from build123d import *

# Parameters (mm, degrees)
SKETCH1_R           = 20
BOSS_EXTRUDE1_DEPTH = 10
SKETCH2_R           = 1
BOSS_EXTRUDE2_DEPTH = 2
SKETCH3_R           = 1
BOSS_EXTRUDE3_DEPTH = 2
FILLET2_R           = 1


with BuildPart() as part:
    # Sketch1 → Boss-Extrude1 (new body)
    with BuildSketch(Plane(origin=(0, 0, 0), x_dir=(0, 0, -1), z_dir=(1, 0, 0))):
        Circle(SKETCH1_R)
    extrude(amount=BOSS_EXTRUDE1_DEPTH)

    # Sketch2 → Boss-Extrude2 (add)
    with BuildSketch(Plane(origin=(10, 0, 0), x_dir=(0, 0, -1), z_dir=(1, 0, 0))):
        Circle(SKETCH2_R)
    extrude(amount=BOSS_EXTRUDE2_DEPTH)

    # Sketch3 → Boss-Extrude3 (add)
    with BuildSketch(Plane.ZY):
        Circle(SKETCH3_R)
    extrude(amount=BOSS_EXTRUDE3_DEPTH)

    # Fillet2
    fillet2_edges = [part.edges().sort_by_distance(p)[0] for p in [
        (0, 0, 20),
        (10, 0, 20),
    ]]
    fillet(fillet2_edges, radius=FILLET2_R)


solid = part.part
Can you work these out from the model? Positions are in its coordinate system, mm. A direction names the side the tool comes from. Round coordinates to 2 decimals unless told otherwise and drop trailing zeros. Order: outer loops, then holes, each group sorted by start corner. A loop starts at its lowest first (then second) coordinate and runs counter-clockwise, first axis right, second up. Notation, with made-up numbers: (-16.75, 18) - (26.25, 18) arc R11 cw to (26.25, 26) - close; hole circle Ø5 at (69.25, 9). An arc over 180 degrees is marked (long way). Answer in a Markdown table with one row per item.
(1) For P1, Ø2, axis at x = 10, y = -10, coming from the +Z side; P2, Ø3, axis at x = 4.5, z = -14.5, coming from the -Y side; P3, Ø6, axis at x = 4.5, z = 7, coming from the -Y side, each with a flat end and sliding along its axis, tell me the tip position at first contact or that it passes through.
From the geometry:
| item | result |
|---|---|
| P1 | stops at z = 17.67 |
| P2 | stops at y = -15.2 |
| P3 | stops at y = -19.6 |
(2) Suppose I cut it at A-A, the plane z = 0. Please give me the cut outline in (x, y), plus the area to 3 significant figures.
From the geometry:
| item | result |
|---|---|
| outline | (-2, -1) - (0, -1) - (0, -19) arc R1 ccw to (1, -20) - (9, -20) arc R1 ccw to (10, -19) - (10, -1) - (12, -1) - (12, 1) - (10, 1) - (10, 19) arc R1 ccw to (9, 20) - (1, 20) arc R1 ccw to (0, 19) - (0, 1) - (-2, 1) - close |
| area | 407 mm2 |
(3) Suppose I cut it at C-C, the plane x = 3.75. Please give me the cut outline in (y, z).
From the geometry:
| item | result |
|---|---|
| outline | circle Ø40 at (0, 0) |
(4) Please list where these lines run through material, in increasing order: L1, parallel to X at y = 16.5, z = -2.5; L2, parallel to Y at x = 0.25, z = -2; L3, parallel to Z at x = 0.25, y = -16. Write a range as from..to.
From the geometry:
| item | result |
|---|---|
| L1 | x = 0..10 |
| L2 | y = -19.56..19.56 |
| L3 | z = -11.43..11.43 |
(5) Which directions (+Z, -Z, +X, -X, +Y, -Y) give clear straight access to the entire face, cutting with the end or side of a thin tool? Please do faces 1 (the face through (-1, -1, 0)), 2 (the face through (4.944, -19.524, 4.336)), 3 (the face through (11, -1, 0)).
From the geometry:
| item | result |
|---|---|
| face 1 | -X |
| face 2 | +X, -X |
| face 3 | +X |
